from build123d import *

# Parameters (mm, degrees)
F0_R     = 5
F1_DEPTH = 7
F3_DEPTH = 7.001


with BuildPart() as f1:
    # F0 (on Top) → F1 (new body)
    with BuildSketch(Plane.XY):
        Circle(F0_R)
    extrude(amount=F1_DEPTH)

    # F2 (on face) → F3 (cut, through all)
    with BuildSketch(Plane.XY.offset(7)):
        with BuildLine():
            Line((1.735315, 1.182659), (-0.247815, 4.092504))
            ThreePointArc((-0.247815, 4.092504), (-3.680977, 1.805659), (-3.387996, -2.309001))
            Line((-3.387996, -2.309001), (1.735315, 1.182659))
        make_face()
        with BuildLine():
            ThreePointArc((-3.387996, -2.309001), (0.334554, -4.086328), (3.718444, -1.727186))
            Line((3.718444, -1.727186), (1.735315, 1.182659))
            Line((1.735315, 1.182659), (-3.387996, -2.309001))
        make_face()
    extrude(amount=-F3_DEPTH, mode=Mode.SUBTRACT)


solid = f1.part
Input: part model. Units: mm. Frame: model coordinates. Round coordinates to 2 decimals unless told otherwise and drop trailing zeros. Write each loop counter-clockwise with the first axis right and the second up, starting at its lowest first coordinate (ties: lowest second). Pieces come first, ordered by that corner, then holes.
1) Cut plane B-B (y = 2.75). Return the cut outline in (x, z), then the cut area to 3 significant figures.
2) Ray query, L1, parallel to X at y = -0.25, z = 3.25; L2, parallel to Y at x = 2.25, z = 2.5; L3, parallel to Y at x = 2, z = 1.75. Return the intervals inside material, ascending.
3) Contact query for flat-ended pins moving along their axis: P1, Ø3, axis at x = 3.5, z = 3, coming from the +Y side; P2, Ø2, axis at x = 3, y = -2.5, coming from the -Z side. Output: stop coordinate, or through.
4) Cut plane C-C (z = 3). Return the cut outline in (x, y).
5) Cut plane A-A (x = -1.5). Return the cut outline in (y, z), then the cut area to 3 significant figures.
Geometry says:
1. outline: (-4.18, 0) - (-3.04, 0) - (-3.04, 7) - (-4.18, 7) - close; (0.67, 0) - (4.18, 0) - (4.18, 7) - (0.67, 7) - close
1. area: 32.5 mm2
2. L1: x = -4.99 to -4.09, 2.71 to 4.99
2. L2: y = -4.47 to -3.43, 0.43 to 4.47
2. L3: y = -4.58 to -3.58, 0.79 to 4.58
3. P1: stops at y = 4.58
3. P2: stops at z = 0
4. outline: circle Ø10 at (0, 0); hole (-3.39, -2.31) arc R4.1 ccw to (3.72, -1.73) - (1.74, 1.18) - (-0.25, 4.09) arc R4.1 ccw to start
5. outline: (-4.77, 0) - (-3.82, 0) - (-3.82, 7) - (-4.77, 7) - close; (3.82, 0) - (4.77, 0) - (4.77, 7) - (3.82, 7) - close
5. area: 13.4 mm2
